Part model, mm, in its own coordinate system. Coordinates: 2 decimals unless noted, no trailing zeros. Order: outer loops, then holes, each group sorted by start corner. A loop starts at its lowest first (then second) coordinate and runs counter-clockwise, first axis right, second up.
Autodesk Inventor part; units mm, degrees
ref_plane "YZ Plane" through (0, 0, 0) normal (1, 0, 0) x (0, 1, 0)
ref_plane "XZ Plane" through (0, 0, 0) normal (0, 1, 0) x (-1, 0, 0)
ref_plane "XY Plane" through (0, 0, 0) normal (0, 0, 1) x (1, 0, 0)
sketch "スケッチ1" plane through (0, 0, 0) normal (0, 0, 1) x (1, 0, 0)
  line L0 (-10, 5) -> (10, 5)
  line L1 (10, 5) -> (10, -5)
  line L2 (10, -5) -> (-10, -5)
  line L3 (-10, -5) -> (-10, 5)
  line L4 (-10, 5) -> (10, -5) construction
  line L5 (10, 5) -> (-10, -5) construction
  point P0 (0, 0)
  dimension "d0" = 20
  dimension "d1" = 10
extrude "押し出し1" add sketch "スケッチ1" along normal blind 1
sketch "スケッチ2" plane through (0, 0, 1) normal (0, 0, 1) x (1, 0, 0)
  line L0 (10, -5) -> (10, 5)
  line L1 (10, 5) -> (-10, 5)
  line L2 (-10, 5) -> (-10, -5)
  point P0 (0, 0)
  point P1 (-5, 0)
  point P2 (5, 0)
  dimension "d4" = 5
  dimension "d5" = 5
  dimension "d6" = 5
  dimension "d7" = 5
hole "穴1" at (-5, 0, 1) at (5, 0, 1) direction (0, 0, -1) diameter 3.2 end through all
properties part number "爪_5" material "アルミニウム 6061"
Q1. Cut at A-A on y = 0. Write the cut outline in (x, z), and give its area (3 significant figures).
Results list:
outline: (-10, 0) - (-6.6, 0) - (-6.6, 1) - (-10, 1) - close; (-3.4, 0) - (3.4, 0) - (3.4, 1) - (-3.4, 1) - close; (6.6, 0) - (10, 0) - (10, 1) - (6.6, 1) - close
area: 13.6 mm2
Q2. Cut at B-B on x = -5. Write the cut outline in (y, z), and give its area (3 significant figures).
Results list:
outline: (-5, 0) - (-1.6, 0) - (-1.6, 1) - (-5, 1) - close; (1.6, 0) - (5, 0) - (5, 1) - (1.6, 1) - close
area: 6.80 mm2
Q3. Cut at D-D on y = 1.25. Write the cut outline in (x, z).
Results list:
outline: (-10, 0) - (-6, 0) - (-6, 1) - (-10, 1) - close; (-4, 0) - (4, 0) - (4, 1) - (-4, 1) - close; (6, 0) - (10, 0) - (10, 1) - (6, 1) - close
Q4. Wall check: line 1 along X through (y, z) = (0, 0.3); line 2 along X through (y, z) = (0.5, 0.6); line 3 along Y through (x, z) = (-5, 0.9). Give the ranges that are in metal, low to high.
Results list:
line 1: x = -10 to -6.6, -3.4 to 3.4, 6.6 to 10
line 2: x = -10 to -6.52, -3.48 to 3.48, 6.52 to 10
line 3: y = -5 to -1.6, 1.6 to 5
Q5. Pin check, flat tip, straight feed: pin 1 Ø3 at (x, y) = (-5, 0) entering from +Z. Stop position of the tip, or through.
Results list:
pin 1: passes through
Q6. Cut at C-C on z = 0.85. Write the cut outline in (x, y), and give its area (3 significant figures).
Results list:
outline: (-10, -5) - (10, -5) - (10, 5) - (-10, 5) - close; hole circle Ø3.2 at (-5, 0); hole circle Ø3.2 at (5, 0)
area: 184 mm2
Q7. Mould opens along X. For faces 1 (the face through (-3.44, 0.35, 0.49)), 2 (the face through (10, 0.1, 0.5)), 3 (the face through (0, 0, 0)) say: pulls with the +X half, pulls with the -X half, needs draft (parallel to the pull), parting line crosses it, or undercut.
Results list:
face 1: undercut
face 2: pulls with the +X half
face 3: needs draft
